For this review, take the finished solid that the model builds, in its own axes (mm). A direction names the side the tool comes from. Coordinates: 2 decimals unless noted, no trailing zeros. Loops run counter-clockwise (first coordinate to the right, second up) from the corner with the lowest first, then second, coordinate; pieces in that order, holes last.
1. Clearance check with flat-ended pins moving along their axes: P1, Ø8, axis at x = 82, z = 49, coming from the +Y side; P2, Ø1.5, axis at x = 70.5, y = 7, coming from the -Z side; P3, Ø4, axis at x = 17, y = 13, coming from the -Z side. State where each tip first meets the part, or that it passes through.
2. Mouldability with a two-part tool opening along Z and no side actions: class faces 5 (the face through (93.4, -6.73, -9.32)), 6 (the face through (12.522, 0.405, -30.625)), 7 (the face through (93.04, 2.931, 106.383)) as pulls with the +Z half, pulls with the -Z half, needs draft (parallel to the pull), parting line crosses it, or undercut.
3. Take a section at D-D, the plane x = 54. State the section outline as (y, z) points.
4. Machinability: for faces 1 (the face through (12.88, -6.73, -9.32)), 2 (the face through (93.04, -28.663, 39.864)), 3 (the face through (93, 30.543, 38)), 4 (the face through (25.4, 0, 5)), which of the approach directions +Z, -Z, +X, -X, +Y, -Y give a long, thin tool a straight path to every point of the face, cutting with its end or side? Answer none if there is none.
5. Take a section at C-C, the plane y = -15. State the section outline as (x, z) points, then the cut area to 3 significant figures.
6. Take a section at B-B, the plane x = 23. State the section outline as (y, z) points, then the cut area to 3 significant figures.
7. To check wall thickness, follow probe 1 along Z at (x, y) = (56, 0); probe 2 along X at (y, z) = (19, 76.5); probe 3 along Z at (x, y) = (100, -3). State the ranges of each line that lie inside material, in increasing order.
8. Take a section at A-A, the plane z = 57.5. State the section outline as (x, y) points.
```python
from build123d import *

# Parameters (mm, degrees)
F0_R      = 30.5430762162
F0_R_2    = 21.9615472454
F1_DEPTH  = 80.518
F3_DEPTH  = 25.4
F5_DEPTH  = 25.4
F6_R      = 18.2049933001
F6_R_2    = 16.9331377315
F7_DEPTH  = 24.384
F8_R      = 17.7079617299
F8_R_2    = 19.0588053324
F9_DEPTH  = 24.638
F10_R     = 11.4627485179
F11_DEPTH = 317.246
F12_R     = 8.4753659895
F13_DEPTH = 402.082


# Not quite as in the source:
# - a feature names something its author has since deleted; it is built from what else it names


with BuildPart() as f1:
    # F0 (on Right) → F1 (new body)
    with BuildSketch(Plane.YZ):
        Circle(F0_R)
        Circle(F0_R_2, mode=Mode.SUBTRACT)
    extrude(amount=F1_DEPTH)

    # F2 (on Right) → F3 (join)
    with BuildSketch(Plane.YZ):
        with BuildLine():
            ThreePointArc((-30.5271036923, -2.0653288811), (1.0640567768, -30.6101895865), (30.6584276259, 0))
            Line((30.6584276259, 0), (30.6584276259, 76.3430893421))
            ThreePointArc((30.6584276259, 76.3430893421), (2.0369783495, 106.5633685136), (-28.2157845795, 77.976256609))
            Line((-28.2157845795, 77.976256609), (-30.5271036923, -2.0653288811))
        make_face()
    extrude(amount=F3_DEPTH)

    # F4 (on face) → F5 (join)
    with BuildSketch(Plane.YZ.offset(80.518)):
        with BuildLine():
            Line((-26.8347635865, 78.6278471351), (-30.5430762162, 0))
            ThreePointArc((-30.5430762162, 0), (0, -30.5430762162), (30.5430762162, 0))
            Line((30.5430762162, 0), (30.5430762162, 77.7075961232))
            ThreePointArc((30.5430762162, 77.7075961232), (2.3069613013, 106.4002056349), (-26.8347635865, 78.6278471351))
        make_face()
    extrude(amount=F5_DEPTH)

    # F6 (on Right) → F7 (join)
    with BuildSketch(Plane.YZ):
        Circle(F6_R)
        with Locations((0, 80.0817832351)):
            Circle(F6_R_2)
    extrude(amount=F7_DEPTH)

    # F8 (on face) → F9 (join)
    with BuildSketch(Plane.YZ.offset(105.918)):
        with Locations((0, 83.1589326262)):
            Circle(F8_R)
        with Locations((0, 4.7338949516)):
            Circle(F8_R_2)
    extrude(amount=-F9_DEPTH)

    # F10 (on face) → F11 (cut)
    with BuildSketch(Plane.YZ.offset(105.918)):
        with Locations((1.8467766198, 77.7075961232)):
            Circle(F10_R)
    extrude(amount=-F11_DEPTH, mode=Mode.SUBTRACT)

    # F12 (on face) → F13 (cut)
    with BuildSketch(Plane.YZ.offset(105.918)):
        with Locations((0, -4.1660955176)):
            Circle(F12_R)
    extrude(amount=-F13_DEPTH, mode=Mode.SUBTRACT)


solid = f1.part
```
Results list:
1. P1: stops at y = 30.54
1. P2: stops at z = -29.9
1. P3: stops at z = -28.6
2. face 5: undercut
2. face 6: pulls with the -Z half
2. face 7: pulls with the +Z half
3. outline: circle Ø61.09 at (0, 0); hole circle Ø43.92 at (0, 0)
4. face 1: +X, -X
4. face 2: +Z, +X, -Y
4. face 3: +Z, -Z, +X, +Y
4. face 4: none
5. outline: (0, -26.69) - (25.4, -26.69) - (25.4, -26.61) - (105.92, -26.61) - (105.92, 100.94) - (80.52, 100.94) - (80.52, 26.61) - (25.4, 26.61) - (25.4, 101.7) - (0, 101.7) - close; hole (25.4, -16.04) - (80.52, -16.04) - (80.52, 16.04) - (25.4, 16.04) - close
5. area: 7,670 mm2
6. outline: (-30.53, -2.07) arc R30.63 ccw to (30.66, 0) - (30.66, 76.34) arc R29.45 ccw to (-28.22, 77.98) - (-30.38, 3.2) arc R30.54 ccw to (-30.51, -1.44) - close; hole circle Ø22.93 at (1.85, 77.71); hole circle Ø16.95 at (0, -4.17)
6. area: 6,830 mm2
7. probe 1: z = -30.54 to -21.96, 21.96 to 30.54
7. probe 2: x = 0 to 25.4, 80.52 to 105.92
7. probe 3: z = -30.4 to -12.09, 3.76 to 67.32, 88.1 to 105.99
8. outline: (0, -28.81) - (25.4, -28.81) - (25.4, 30.66) - (0, 30.66) - close; (80.52, -27.83) - (105.92, -27.83) - (105.92, 30.54) - (80.52, 30.54) - close
